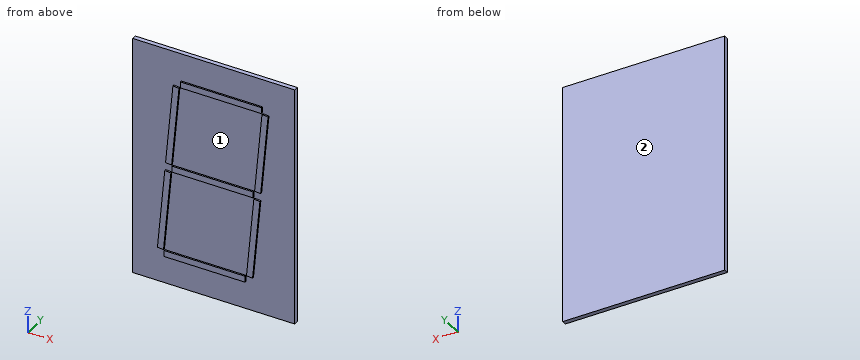
```python
from build123d import *

# Parameters (mm, degrees)
F0_W     = 100.000007
F0_H     = 7.500015
F1_DEPTH = 2
F0_W_2   = 100
F0_H_2   = 7.5
F0_W_3   = 100.000004
F2_W     = 200
F2_H     = 295
F3_DEPTH = 5.5


with BuildPart() as f1:
    # F0 (on Front) → F1 (new body)
    with BuildSketch(Plane.XZ):
        with Locations((10.0000135, 109.4999925)):
            Rectangle(F0_W, F0_H)
    extrude(amount=F1_DEPTH)



with BuildPart() as f1b:
    # F0 (on Front) → F1, piece 2 (new body)
    with BuildSketch(Plane.XZ):
        Polygon((-49.156019, 105.224884), (-58.250597, 5.639297), (-50.781679, 4.957199), (-41.687101, 104.542786), align=None)
    extrude(amount=F1_DEPTH)


with BuildPart() as f1c:
    # F0 (on Front) → F1, piece 3 (new body)
    with BuildSketch(Plane.XZ):
        Polygon((60.812838, 104.883835), (51.718248, 5.298248), (59.187182, 4.61615), (68.281756, 104.201736), align=None)
    extrude(amount=F1_DEPTH)


with BuildPart() as f1d:
    # F0 (on Front) → F1, piece 4 (new body)
    with BuildSketch(Plane.XZ):
        with Locations((2e-06, 1.5e-05)):
            Rectangle(F0_W_2, F0_H_2)
    extrude(amount=F1_DEPTH)


with BuildPart() as f1e:
    # F0 (on Front) → F1, piece 5 (new body)
    with BuildSketch(Plane.XZ):
        Polygon((-59.18717, -4.61615), (-68.28175, -104.20174), (-60.81283, -104.883835), (-51.718252, -5.298248), align=None)
    extrude(amount=F1_DEPTH)


with BuildPart() as f1f:
    # F0 (on Front) → F1, piece 6 (new body)
    with BuildSketch(Plane.XZ):
        with Locations((-10, -109.499992)):
            Rectangle(F0_W_3, F0_H_2)
    extrude(amount=F1_DEPTH)


with BuildPart() as f1g:
    # F0 (on Front) → F1, piece 7 (new body)
    with BuildSketch(Plane.XZ):
        Polygon((50.781679, -4.957199), (41.687105, -104.542789), (49.156023, -105.22488), (58.250597, -5.639297), align=None)
    extrude(amount=F1_DEPTH)


with BuildPart() as f1_1:
    add(f1.part)

    add(f1b.part)  # F3 merges F1b

    add(f1c.part)  # F3 merges F1c

    add(f1d.part)  # F3 merges F1d

    add(f1e.part)  # F3 merges F1e

    add(f1f.part)  # F3 merges F1f

    add(f1g.part)  # F3 merges F1g
    # F2 (on Front) → F3 (join)
    with BuildSketch(Plane.XZ):
        with Locations((2e-06, 0)):
            Rectangle(F2_W, F2_H)
    extrude(amount=-F3_DEPTH)


solid = f1_1.part
```
Here's how the part is built. I have some questions about the finished solid (model axes, mm). Face numbers are marked on the shaded views. Give positions to 0.01 mm unless a question says otherwise; leave off trailing zeros. Loops run counter-clockwise (first coordinate to the right, second up) from the corner with the lowest first, then second, coordinate; pieces in that order, holes last. Notation, with made-up numbers: M 32,31 L 66,31 A20 cw 66,46 Z; hole C 52.5,14.5 d10. An arc over 180 degrees is marked long. Return JSON: item names as keys, results as strings.
Item 1: I'm going to push flat-ended pins straight in: pin 1 Ø0.6 at (y, z) = (-1, -108) entering from +X; pin 2 Ø1 at (y, z) = (-1, 1.5) entering from -X; pin 3 Ø1 at (x, z) = (68.5, 67) entering from -Y; pin 4 Ø3 at (y, z) = (-0.5, 52.5) entering from +X. Where does each tip first touch, or does it pass through?
A:
{"pin 1": "stops at x = 40", "pin 2": "stops at x = -50", "pin 3": "stops at y = 0", "pin 4": "stops at x = 100"}
Item 2: Imagine slicing it at B-B on z = -116.5. List the corners of the cut face in (x, y) for me, then the cut area to 3 significant figures.
A:
{"outline": "M -100,0 L 100,0 L 100,5.5 L -100,5.5 Z", "area": "1,100 mm^2"}
Item 3: Imagine slicing it at A-A on x = -33.5. List the corners of the cut face in (y, z) for me.
A:
{"outline": "M -2,-113.25 L 0,-113.25 L 0,-147.5 L 5.5,-147.5 L 5.5,147.5 L 0,147.5 L 0,113.25 L -2,113.25 L -2,105.75 L 0,105.75 L 0,3.75 L -2,3.75 L -2,-3.75 L 0,-3.75 L 0,-105.75 L -2,-105.75 Z"}
Item 4: Imagine slicing it at C-C on z = -44. List the corners of the cut face in (x, y) for me, then the cut area to 3 significant figures.
A:
{"outline": "M -100,0 L -62.78,0 L -62.78,-2 L -55.25,-2 L -55.25,0 L 47.22,0 L 47.22,-2 L 54.75,-2 L 54.75,0 L 100,0 L 100,5.5 L -100,5.5 Z", "area": "1,130 mm^2"}
Item 5: Please list where these lines run through material, in increasing order: line 1 (Z direction, x = 18.5, y = -1.25); line 2 (Y direction, x = 58, z = -94); line 3 (X direction, y = -1.5, z = -72).
A:
{"line 1": "z = -113.25 to -105.75, -3.75 to 3.75, 105.75 to 113.25", "line 2": "y = 0 to 5.5", "line 3": "x = -65.34 to -57.81, 44.66 to 52.19"}
Item 6: Thinking about a two-plate mould opening in X: for the marked faces 1 and 2, which applies, released by +X, released by -X, zero draft, split by the parting line, or undercut?
A:
{"face 1": "undercut", "face 2": "zero draft"}
Item 7: Imagine slicing it at D-D on x = -83. List the corners of the cut face in (y, z) for me.
A:
{"outline": "M 0,-147.5 L 5.5,-147.5 L 5.5,147.5 L 0,147.5 Z"}
